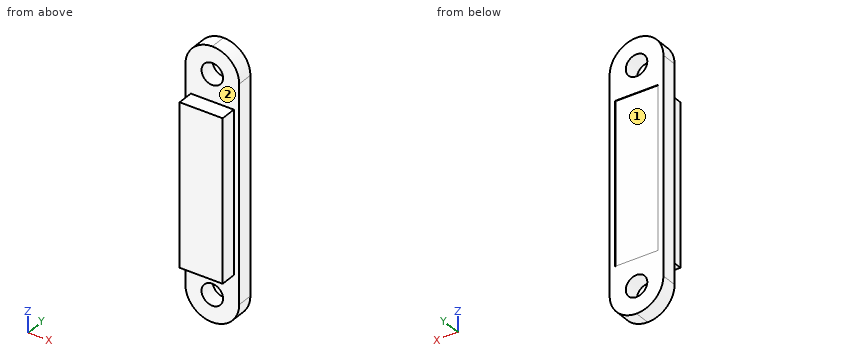
Autodesk Inventor part; units mm, degrees
ref_plane "YZ Plane" through (0, 0, 0) normal (1, 0, 0) x (0, 1, 0)
ref_plane "XZ Plane" through (0, 0, 0) normal (0, 1, 0) x (-1, 0, 0)
ref_plane "XY Plane" through (0, 0, 0) normal (0, 0, 1) x (1, 0, 0)
sketch "Эскиз1" plane through (0, 0, 0) normal (0, 1, 0) x (-1, 0, 0)
  line L0 (-11.1966, 15.641) -> (-1.1966, 15.641)
  line L1 (-1.1966, 15.641) -> (-1.1966, -34.359)
  line L2 (-1.1966, -34.359) -> (-11.1966, -34.359)
  line L3 (-11.1966, -34.359) -> (-11.1966, 15.641)
  point P0 (0, 0)
  dimension "d0" = 50
  dimension "d1" = 10
extrude "Выдавливание1" add sketch "Эскиз1" along normal blind 3
fillet "Сопряжение1" radius 5 2 edges at (11.1966, 1.5, -34.359) (1.1966, 1.5, -34.359)
fillet "Сопряжение2" radius 5 2 edges at (11.1966, 1.5, 15.641) (1.1966, 1.5, 15.641)
sketch "Эскиз2" plane through (0, 3, 0) normal (0, 1, 0) x (1, 0, 0)
  line L0 (2.1966, 24.359) -> (10.1966, 24.359)
  line L1 (10.1966, 24.359) -> (10.1966, -5.641)
  line L2 (10.1966, -5.641) -> (2.1966, -5.641)
  line L3 (2.1966, -5.641) -> (2.1966, 24.359)
  arc A0 (11.1966, 29.359) -> (1.1966, 29.359) centre (6.1966, 29.359) ccw
  arc A1 (1.1966, -10.641) -> (11.1966, -10.641) centre (6.1966, -10.641) ccw
  line L4 (11.1966, -10.641) -> (11.1966, 29.359)
  line L5 (1.1966, 29.359) -> (1.1966, -10.641)
  point P0 (0, 0)
  point P1 (6.1966, 34.359)
  point P2 (6.1966, 24.359)
  point P3 (6.1966, -15.641)
  point P4 (6.1966, -5.641)
  dimension "d6" = 10
  dimension "d7" = 10
  dimension "d8" = 1
  dimension "d9" = 1
extrude "Выдавливание2" cut sketch "Эскиз2" against normal blind 0.1 contours L0 L1 L2 L3
sketch "Эскиз3" plane through (0, 3, 0) normal (0, 1, 0) x (1, 0, 0)
  circle A0 centre (23.3894, 111.2567) radius 1
  circle A1 centre (6.1966, 29.359) radius 2
  arc A2 (11.1966, 29.359) -> (1.1966, 29.359) centre (6.1966, 29.359) ccw
  circle A3 centre (6.1966, -10.641) radius 2
  arc A4 (1.1966, -10.641) -> (11.1966, -10.641) centre (6.1966, -10.641) ccw
  point P0 (0, 0)
  point P1 (6.1966, 34.359)
  point P2 (6.1966, -15.641)
  dimension "d12" = 2
  dimension "d13" = 4
  dimension "d14" = 5
  dimension "d15" = 4
extrude "Выдавливание3" cut sketch "Эскиз3" against normal blind 10 contours A1 | A3
sketch "Эскиз4" plane through (0, 0, 0) normal (0, -1, 0) x (1, 0, 0)
  line L0 (10.1966, 5.641) -> (2.1966, 5.641)
  line L1 (2.1966, 5.641) -> (2.1966, -24.359)
  line L2 (10.1966, 5.641) -> (2.1966, 5.641)
  line L3 (2.1966, 5.641) -> (2.1966, -24.359)
  line L4 (2.1966, -24.359) -> (10.1966, -24.359)
  line L5 (10.1966, -24.359) -> (10.1966, 5.641)
  point P0 (0, 0)
extrude "Выдавливание4" add sketch "Эскиз4" along normal blind 3
properties part number "магнит 2" material "Сталь"
For this review, take the finished solid that the model builds, in its own axes (mm). Face numbers are marked on the shaded views. Round coordinates to 2 decimals unless told otherwise and drop trailing zeros. Loops run counter-clockwise (first coordinate to the right, second up) from the corner with the lowest first, then second, coordinate; pieces in that order, holes last.
(1) We need section B-B (z = -28). Give the boundary of the cut face in (x, y), plus the area to 3 significant figures.
Returned:
outline: (1.2, 0) - (4.73, 0) - (4.73, 3) - (1.2, 3) - close; (7.66, 0) - (11.2, 0) - (11.2, 3) - (7.66, 3) - close
area: 21.2 mm2
(2) We need section A-A (x = 5.75). Give the boundary of the cut face in (y, z).
Returned:
outline: (-3, -24.36) - (0, -24.36) - (0, -27.41) - (3, -27.41) - (3, -24.36) - (2.9, -24.36) - (2.9, 5.64) - (3, 5.64) - (3, 8.69) - (0, 8.69) - (0, 5.64) - (-3, 5.64) - close; (0, -34.34) - (3, -34.34) - (3, -31.31) - (0, -31.31) - close; (0, 12.59) - (3, 12.59) - (3, 15.62) - (0, 15.62) - close
(3) Clearance check with flat-ended pins moving along their axes: P1, Ø0.9, axis at y = -1, z = -8, coming from the +X side; P2, Ø2.5, axis at x = 7.5, y = -1.5, coming from the +Z side; P3, Ø1.5, axis at y = -2, z = -12.5, coming from the -X side; P4, Ø5, axis at x = 9.5, z = 4, coming from the +Y side. State where each tip first meets the part, or that it passes through.
Returned:
P1: stops at x = 10.2
P2: stops at z = 5.64
P3: stops at x = 2.2
P4: stops at y = 3
(4) We need section C-C (y = 1.2). State how many separate pieces and enclosed holes the cut face has, plus the area to 3 significant figures.
Returned:
separate pieces: 1
enclosed holes: 2
area: 453 mm2
(5) We need section D-D (z = -14.5). Give the boundary of the cut face in (x, y), plus the area to 3 significant figures.
Returned:
outline: (1.2, 0) - (2.2, 0) - (2.2, -3) - (10.2, -3) - (10.2, 0) - (11.2, 0) - (11.2, 3) - (10.2, 3) - (10.2, 2.9) - (2.2, 2.9) - (2.2, 3) - (1.2, 3) - close
area: 53.2 mm2
(6) Mouldability with a two-part tool opening along Z and no side actions: class the marked faces 1 and 2 as released by +Z, released by -Z, zero draft, split by the parting line, or undercut.
Returned:
face 1: undercut
face 2: zero draft
(7) Wall thickness on line 1 along Z through (x, y) = (10, -2.15); line 2 along Y through (x, z) = (1.75, 0.5); line 3 along Y through (x, z) = (3, -11): over which ranges is each line inside the solid? List them lowest first.
Returned:
line 1: z = -24.36 to 5.64
line 2: y = 0 to 3
line 3: y = -3 to 2.9
